Part model, mm, in its own coordinate system. A direction names the side the tool comes from. Coordinates: 2 decimals unless noted, no trailing zeros. Order: outer loops, then holes, each group sorted by start corner. A loop starts at its lowest first (then second) coordinate and runs counter-clockwise, first axis right, second up. Notation, with made-up numbers: M -14.5,-26.75 L -7.5,-26.75 A30 ccw -7.5,1.25 Z; hole C 0.5,9.25 d9. An arc over 180 degrees is marked long. Write item = value, one per line. Start each with the question number.
from build123d import *
from build123d.topology import SkipClean

# Parameters (mm, degrees)
ESQUISSE1_R                  = 10
BOSS_EXTRU_1_DEPTH           = 30
ESQUISSE2_R                  = 5.752589483
BOSS_EXTRU_2_DEPTH           = 30
BOSS_EXTRU_3_DEPTH           = 15
ENL_V_MAT_EXTRU_1_DEPTH      = 77.645000637
ENL_V_MAT_EXTRU_1_DEPTH_BACK = 77.645000637
ESQUISSE4_R                  = 2


with BuildPart() as part:
    # Esquisse1 → Boss.-Extru.1 (new body)
    with BuildSketch(Plane.XY):
        Circle(ESQUISSE1_R)
    extrude(amount=BOSS_EXTRU_1_DEPTH)

    # Esquisse2 → Boss.-Extru.2 (add)
    with BuildSketch(Plane.XY.offset(30)):
        Circle(ESQUISSE2_R)
    extrude(amount=BOSS_EXTRU_2_DEPTH)

    # Esquisse3 → Boss.-Extru.3 (add)
    with SkipClean():  # the faces are left unmerged after this step: merging them gives an invalid solid
        with BuildSketch(Plane.XY.offset(60)):
            with BuildLine():
                Line((-2.225224852, 5.304777104), (-2.225224852, -5.304777104))
                ThreePointArc((-2.225224852, -5.304777104), (-5.752589483, 0), (-2.225224852, 5.304777104))
            make_face()
            with BuildLine():
                Line((2.225224852, 5.304777104), (2.225224852, -5.304777104))
                ThreePointArc((2.225224852, -5.304777104), (5.752589483, 0), (2.225224852, 5.304777104))
            make_face()
        extrude(amount=BOSS_EXTRU_3_DEPTH)

    # Esquisse4 → Enlèv. mat.-Extru.1 (cut, two sides: drawn at the far end of the back side and taken through both)
    with SkipClean():  # the faces are left unmerged after this step: merging them gives an invalid solid
        with BuildSketch(Plane.ZY.offset(-2.225224852).offset(-ENL_V_MAT_EXTRU_1_DEPTH_BACK)):
            with Locations((67.284392663, 0)):
                Circle(ESQUISSE4_R)
        extrude(amount=ENL_V_MAT_EXTRU_1_DEPTH + ENL_V_MAT_EXTRU_1_DEPTH_BACK, mode=Mode.SUBTRACT)


solid = part.part
Item 1: Pull direction Y, two halves, no side cores. Call faces 3 (the cylindrical face through (-2.17, -9.76, 14.79)), 4 (the cylindrical face through (-3.966, 0.088, 65.286)), 5 (the flat face through (4.3, -4.3, 30)): pulls with the +Y half, pulls with the -Y half, needs draft (parallel to the pull), parting line crosses it, or undercut.
Item 2: Cut at D-D, the plane y = -3. Write the cut outline in (x, z), and give its area (3 significant figures).
Item 3: Cut at C-C, the plane z = 35.5. Write the cut outline in (x, y), and give its area (3 significant figures).
Item 4: Wall check: line 1 along Z through (x, y) = (-4.5, 0); line 2 along Z through (x, y) = (8, -3.5); line 3 along Z through (x, y) = (-1, 4.75). Give the ranges that are in metal, low to high. Write a range as [from, to].
Item 5: Cut at B-B, the plane x = 0. Write the cut outline in (y, z).
Item 6: Cut at A-A, the plane y = 0. Write the cut outline in (x, z).
Item 7: Flat gauge pins, fed straight in: pin 1 (3 mm diameter, centred on y = 0, z = 67.28, fed in from +X); pin 2 (4 mm diameter, centred on x = -6.5, z = 8, fed in from -Y); pin 3 (2 mm diameter, centred on y = -4, z = 59, fed in from +X); pin 4 (1 mm diameter, centred on x = 2.5, z = 28.5, fed in from -Y). Where does each tip first touch, or does it go through?
Item 8: 3-axis set-ups, long thin cutter, end or side, ignore diameter. For faces 1 (the flat face through (0, 0, 0)), 2 (the flat face through (-2.225, 1.3, 69.1)): which of +Z, -Z, +X, -X, +Y, -Y reach the whole face in a straight line?
Filled sheet:
q1.face_3 = parting line crosses it
q1.face_4 = undercut
q1.face_5 = needs draft
q2.outline = M -9.54,0 L 9.54,0 L 9.54,30 L 4.91,30 L 4.91,75 L 2.23,75 L 2.23,60 L -2.23,60 L -2.23,75 L -4.91,75 L -4.91,30 L -9.54,30 Z
q2.area = 947 mm2
q3.outline = C 0,0 d11.51
q3.area = 104 mm2
q4.line_1 = [0, 65.28], [69.28, 75]
q4.line_2 = [0, 30]
q4.line_3 = [0, 60]
q5.outline = M -10,0 L 10,0 L 10,30 L 5.75,30 L 5.75,60 L -5.75,60 L -5.75,30 L -10,30 Z
q6.outline = M -10,0 L 10,0 L 10,30 L 5.75,30 L 5.75,65.28 L 2.23,65.28 L 2.23,60 L -2.23,60 L -2.23,65.28 L -5.75,65.28 L -5.75,30 L -10,30 Z; M -5.75,69.28 L -2.23,69.28 L -2.23,75 L -5.75,75 Z; M 2.23,69.28 L 5.75,69.28 L 5.75,75 L 2.23,75 Z
q7.pin_1 = through
q7.pin_2 = -8.93
q7.pin_3 = 4.91
q7.pin_4 = -9.8
q8.face_1 = -Z, +X, -X, +Y, -Y
q8.face_2 = +Z, +Y, -Y
